Part model, mm, in its own coordinate system. A direction names the side the tool comes from. Coordinates: 2 decimals unless noted, no trailing zeros. Write each loop counter-clockwise with the first axis right and the second up, starting at its lowest first coordinate (ties: lowest second). Pieces come first, ordered by that corner, then holes. Notation, with made-up numbers: (-21, 65) -> (-2, 65) arc R23 ccw to (-2, 81) -> close; hole circle Ø1 at (68.25, 23.25). An arc over 180 degrees is marked (long way). Write item = value, one per line.
from build123d import *

# Parameters (mm, degrees)
ESQUISSE1_W              = 40
ESQUISSE1_H              = 40
BOSS_EXTRU_1_DEPTH       = 50
ESQUISSE2_R              = 5
ENL_V_MAT_EXTRU_1_DEPTH  = 41
ESQUISSE3_R              = 5
ENL_V_MAT_EXTRU_2_DEPTH  = 41
ESQUISSE4_W              = 22
ESQUISSE4_H              = 14
ENL_V_MAT_EXTRU_3_DEPTH  = 29
ESQUISSE5_W              = 14
ESQUISSE5_H              = 20
ENL_V_MAT_EXTRU_4_DEPTH  = 29
ESQUISSE6_W              = 20
ESQUISSE6_H              = 14
ENL_V_MAT_EXTRU_5_DEPTH  = 24
ESQUISSE7_W              = 14
ESQUISSE7_H              = 22
ENL_V_MAT_EXTRU_6_DEPTH  = 24
ESQUISSE10_R             = 11
ENL_V_MAT_EXTRU_9_DEPTH  = 7
ESQUISSE11_R             = 12.5
ENL_V_MAT_EXTRU_10_DEPTH = 1.5
ESQUISSE14_R             = 11
ENL_V_MAT_EXTRU_11_DEPTH = 7
ESQUISSE15_R             = 12.5
ENL_V_MAT_EXTRU_12_DEPTH = 1.5
ESQUISSE16_W             = 40
ESQUISSE16_H             = 40
BOSS_EXTRU_2_DEPTH       = 7
ESQUISSE17_R             = 2.25
ENL_V_MAT_EXTRU_13_DEPTH = 15
ESQUISSE18_W             = 3.5
ESQUISSE18_H             = 7.5
ENL_V_MAT_EXTRU_14_DEPTH = 12
ESQUISSE19_W             = 7.5
ESQUISSE19_H             = 3.5
ENL_V_MAT_EXTRU_15_DEPTH = 12


with BuildPart() as part:
    # Esquisse1 → Boss.-Extru.1 (new body)
    with BuildSketch(Plane.XY):
        with Locations((-20, 20)):
            Rectangle(ESQUISSE1_W, ESQUISSE1_H)
    extrude(amount=BOSS_EXTRU_1_DEPTH)

    # Esquisse2 → Enlèv. mat.-Extru.1 (cut, through all)
    with BuildSketch(Plane(origin=(0, 40, 0), x_dir=(1, 0, 0), z_dir=(0, 1, 0))):
        with Locations(Location((-20, -15, 0), (0, 0, 270))):  # turned: the seam where the file's is
            Circle(ESQUISSE2_R)
    extrude(amount=-ENL_V_MAT_EXTRU_1_DEPTH, mode=Mode.SUBTRACT)

    # Esquisse3 → Enlèv. mat.-Extru.2 (cut, through all)
    with BuildSketch(Plane.ZY.offset(40)):
        with Locations((35, 20)):
            Circle(ESQUISSE3_R)
    extrude(amount=-ENL_V_MAT_EXTRU_2_DEPTH, mode=Mode.SUBTRACT)

    # Esquisse4 → Enlèv. mat.-Extru.3 (cut)
    with BuildSketch(Plane.ZY.offset(40)):
        with Locations((11, 20)):
            Rectangle(ESQUISSE4_W, ESQUISSE4_H)
    extrude(amount=-ENL_V_MAT_EXTRU_3_DEPTH, mode=Mode.SUBTRACT)

    # Esquisse5 → Enlèv. mat.-Extru.4 (cut)
    with BuildSketch(Plane.XZ):
        with Locations((-20, 35)):
            Rectangle(ESQUISSE5_W, ESQUISSE5_H)
    extrude(amount=-ENL_V_MAT_EXTRU_4_DEPTH, mode=Mode.SUBTRACT)

    # Esquisse6 → Enlèv. mat.-Extru.5 (cut)
    with BuildSketch(Plane(origin=(0, 0, 0), x_dir=(0, 0, -1), z_dir=(1, 0, 0))):
        with Locations((-15, 20)):
            Rectangle(ESQUISSE6_W, ESQUISSE6_H)
    extrude(amount=-ENL_V_MAT_EXTRU_5_DEPTH, mode=Mode.SUBTRACT)

    # Esquisse7 → Enlèv. mat.-Extru.6 (cut)
    with BuildSketch(Plane(origin=(0, 40, 0), x_dir=(1, 0, 0), z_dir=(0, 1, 0))):
        with Locations((-20, -39)):
            Rectangle(ESQUISSE7_W, ESQUISSE7_H)
    extrude(amount=-ENL_V_MAT_EXTRU_6_DEPTH, mode=Mode.SUBTRACT)

    # Esquisse10 → Enlèv. mat.-Extru.9 (cut)
    with BuildSketch(Plane(origin=(0, 40, 0), x_dir=(1, 0, 0), z_dir=(0, 1, 0))):
        with Locations(Location((-20, -15, 0), (0, 0, 270))):  # turned: the seam where the file's is
            Circle(ESQUISSE10_R)
    extrude(amount=-ENL_V_MAT_EXTRU_9_DEPTH, mode=Mode.SUBTRACT)

    # Esquisse11 → Enlèv. mat.-Extru.10 (cut)
    with BuildSketch(Plane(origin=(0, 40, 0), x_dir=(1, 0, 0), z_dir=(0, 1, 0))):
        with Locations(Location((-20, -15, 0), (0, 0, 270))):  # turned: the seam where the file's is
            Circle(ESQUISSE11_R)
    extrude(amount=-ENL_V_MAT_EXTRU_10_DEPTH, mode=Mode.SUBTRACT)

    # Esquisse14 → Enlèv. mat.-Extru.11 (cut)
    with BuildSketch(Plane.ZY.offset(40)):
        with Locations((35, 20)):
            Circle(ESQUISSE14_R)
    extrude(amount=-ENL_V_MAT_EXTRU_11_DEPTH, mode=Mode.SUBTRACT)

    # Esquisse15 → Enlèv. mat.-Extru.12 (cut)
    with BuildSketch(Plane.ZY.offset(40)):
        with Locations((35, 20)):
            Circle(ESQUISSE15_R)
    extrude(amount=-ENL_V_MAT_EXTRU_12_DEPTH, mode=Mode.SUBTRACT)

    # Esquisse16 → Boss.-Extru.2 (add)
    with BuildSketch(Plane(origin=(0, 0, 0), x_dir=(-1, 0, 0), z_dir=(0, 0, -1))):
        with Locations((20, 20)):
            Rectangle(ESQUISSE16_W, ESQUISSE16_H)
    extrude(amount=BOSS_EXTRU_2_DEPTH)

    # Esquisse17 → Enlèv. mat.-Extru.13 (cut)
    with BuildSketch(Plane(origin=(0, 0, -7), x_dir=(-1, 0, 0), z_dir=(0, 0, -1))):
        with Locations((7.5, 30)):
            Circle(ESQUISSE17_R)
        with Locations((30, 7.5)):
            Circle(ESQUISSE17_R)
    extrude(amount=-ENL_V_MAT_EXTRU_13_DEPTH, mode=Mode.SUBTRACT)

    # Esquisse18 → Enlèv. mat.-Extru.14 (cut)
    with BuildSketch(Plane(origin=(0, 0, 0), x_dir=(0, 0, -1), z_dir=(1, 0, 0))):
        with Locations((1.25, 30)):
            Rectangle(ESQUISSE18_W, ESQUISSE18_H)
    extrude(amount=-ENL_V_MAT_EXTRU_14_DEPTH, mode=Mode.SUBTRACT)

    # Esquisse19 → Enlèv. mat.-Extru.15 (cut)
    with BuildSketch(Plane.XZ):
        with Locations((-30, -1.25)):
            Rectangle(ESQUISSE19_W, ESQUISSE19_H)
    extrude(amount=-ENL_V_MAT_EXTRU_15_DEPTH, mode=Mode.SUBTRACT)


solid = part.part
Q1. Mould opens along Z. For faces 1 (the face through (-20, 0, 22)), 2 (the face through (-27, 20.3, 40.5)), 3 (the face through (-30, 8, 8)), 4 (the face through (-20, 35, 28)) say: released by +Z, released by -Z, zero draft, split by the parting line, or undercut.
Model answer:
face_1 = zero draft
face_2 = undercut
face_3 = released by -Z
face_4 = released by +Z
Q2. Which spindle directions (+Z, -Z, +X, -X, +Y, -Y) get a long thin tool onto all of the face, cutting with end or side? Do faces 5 (the face through (-30.74, 35.79, 12.62)), 6 (the face through (-31.21, 9.397, 4.198)), 7 (the face through (-32, 20, 22)). Say none if no direction does.
Model answer:
face_5 = +Y
face_6 = -Z
face_7 = +X, -X
Q3. Saw through at C-C on x = -3. Give the cut face in (y, z).
Model answer:
outline = (0, -7) -> (40, -7) -> (40, 50) -> (0, 50) -> close; hole (13, 5) -> (27, 5) -> (27, 25) -> (13, 25) -> close; hole circle Ø10 at (20, 35); hole (26.25, -3) -> (33.75, -3) -> (33.75, 0.5) -> (26.25, 0.5) -> close
Q4. Saw through at A-A on y = 20. Count the separate pieces of the cut face and the enclosed holes in it, and give its area (4 significant figures).
Model answer:
separate_pieces = 5
enclosed_holes = 0
area = 684.5 mm²
Q5. Saw through at B-B on z = 15. Give the cut face in (x, y), and give its area (4 significant figures).
Model answer:
outline = (-40, 0) -> (-25, 0) -> (-25, 13) -> (-40, 13) -> close; (-40, 27) -> (-25, 27) -> (-25, 33) -> (-31, 33) -> (-31, 38.5) -> (-32.5, 38.5) -> (-32.5, 40) -> (-40, 40) -> close; (-15, 0) -> (0, 0) -> (0, 13) -> (-15, 13) -> close; (-15, 27) -> (0, 27) -> (0, 40) -> (-7.5, 40) -> (-7.5, 38.5) -> (-9, 38.5) -> (-9, 33) -> (-15, 33) -> close
area = 691.5 mm²
Q6. Probe line 1 (Y direction, x = -3, z = -1.5); line 2 (X direction, y = 13.5, z = 27); line 3 (Z direction, x = -3, y = 24.5). List the from-to ranges inside material, lowest first. Write a range as from..to.
Model answer:
line_1 = 0..26.25, 33.75..40
line_2 = -33..-27, -13..0
line_3 = -7..5, 25..32.82, 37.18..50
Q7. Pin check, flat tips, straight feed: pin 1 (2.5 mm diameter, centred on x = -19.5, z = 48, fed in from +Y); pin 2 (9 mm diameter, centred on x = -21, y = 36.5, fed in from +Z); pin 3 (20 mm diameter, centred on y = 20, z = 35, fed in from -X). Stop position of each tip, or through.
Model answer:
pin_1 = 16
pin_2 = 28
pin_3 = -33
